```python
from build123d import *

# Parameters (mm, degrees)
F0_W     = 36.2055785954
F0_H     = 36.4281870425
F1_DEPTH = 25.4
F2_R     = 5.9545672291
F3_DEPTH = 101.6
F4_R     = 3.175
F5_DEPTH = 36.4291870425


with BuildPart() as f1:
    # F0 (on Top) → F1 (new body)
    with BuildSketch(Plane.XY):
        with Locations((18.1027892977, 19.5768494159)):
            Rectangle(F0_W, F0_H)
    extrude(amount=F1_DEPTH)

    # F2 (on face) → F3 (join)
    with BuildSketch(Plane.XY.offset(25.4)):
        with Locations((16.946144402, 22.8772908449)):
            Circle(F2_R)
    extrude(amount=F3_DEPTH)

    # F4 (on face) → F5 (cut, through all)
    with BuildSketch(Plane.XZ.offset(-1.3627558947)):
        with Locations((19.3670187145, 18.4601526707)):
            Circle(F4_R)
    extrude(amount=-F5_DEPTH, mode=Mode.SUBTRACT)


solid = f1.part
```
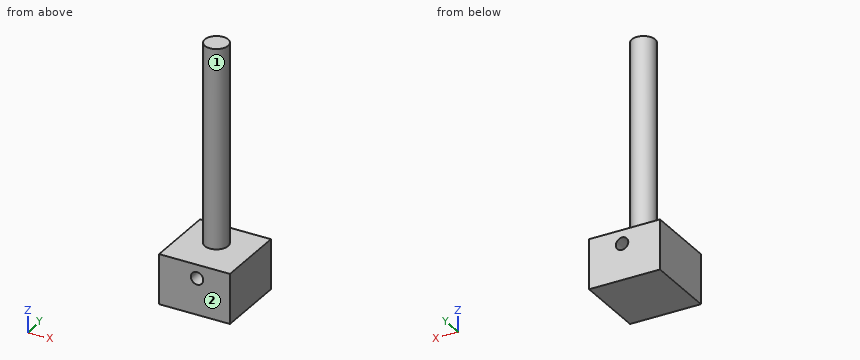
Input: part model. Units: mm. Frame: model coordinates. Face numbers are marked on the shaded views. A direction names the side the tool comes from. Coordinates: 2 decimals unless noted, no trailing zeros. Order: outer loops, then holes, each group sorted by start corner. A loop starts at its lowest first (then second) coordinate and runs counter-clockwise, first axis right, second up. Notation, with made-up numbers: (-18, 21) - (20, 21) arc R34 ccw to (20, 54) - close; hole circle Ø6 at (-34, -16). An arc over 180 degrees is marked (long way). Return JSON: item names as keys, results as strings.
Q1. First-contact query: pin 1 (3 mm diameter, centred on y = 27, z = 80, fed in from +X); pin 2 (4 mm diameter, centred on x = 21, z = 90, fed in from +Y); pin 3 (12 mm diameter, centred on y = 23, z = 81.5, fed in from -X); pin 4 (8 mm diameter, centred on x = 28, z = 75, fed in from -Y). Flat tips, straight axial feed; report the tip coordinate or a pass-through.
The answers:
{"pin 1": "stops at x = 22.29", "pin 2": "stops at y = 28.47", "pin 3": "stops at x = 10.99", "pin 4": "passes through"}
Q2. Cut plane C-C (x = 12.5). Return loops of the section in (y, z), then the cut area to 3 significant figures.
The answers:
{"outline": "(1.36, 0) - (37.79, 0) - (37.79, 25.4) - (26.84, 25.4) - (26.84, 127) - (18.92, 127) - (18.92, 25.4) - (1.36, 25.4) - close", "area": "1,730 mm2"}
Q3. Access query for the marked faces 1 and 2. Directions: +Z, -Z, +X, -X, +Y, -Y. A direction counts if a zero-diameter tool reaches every point of the face in a straight line with its end or side. Return the directions, or none.
The answers:
{"face 1": "+Z", "face 2": "+Z, -Z, +X, -X, -Y"}
Q4. Cut plane D-D (y = 35.5). Return loops of the section in (x, z) (3 decimals).
The answers:
{"outline": "(0, 0) - (36.206, 0) - (36.206, 25.4) - (0, 25.4) - close; hole circle Ø6.35 at (19.367, 18.46)"}
Q5. Cut plane A-A (x = 18). Return loops of the section in (y, z), then the cut area to 3 significant figures.
The answers:
{"outline": "(1.36, 0) - (37.79, 0) - (37.79, 15.59) - (1.36, 15.59) - close; (1.36, 21.33) - (37.79, 21.33) - (37.79, 25.4) - (28.74, 25.4) - (28.74, 127) - (17.02, 127) - (17.02, 25.4) - (1.36, 25.4) - close", "area": "1,910 mm2"}
Q6. Cut plane B-B (y = 20.5). Return loops of the section in (x, z) (3 decimals), then the cut area to 3 significant figures.
The answers:
{"outline": "(0, 0) - (36.206, 0) - (36.206, 25.4) - (22.406, 25.4) - (22.406, 127) - (11.487, 127) - (11.487, 25.4) - (0, 25.4) - close; hole circle Ø6.35 at (19.367, 18.46)", "area": "2,000 mm2"}
Q7. Ray query, probe 1 along Z at (x, y) = (19.5, 23); probe 2 along X at (y, z) = (23, 56); probe 3 along Z at (x, y) = (27.5, 29). Return the intervals inside material, ascending.
The answers:
{"probe 1": "z = 0 to 15.29, 21.63 to 127", "probe 2": "x = 10.99 to 22.9", "probe 3": "z = 0 to 25.4"}
